Source: CAD feature listing. Evaluate the final solid. Frame: model axes, mm. A direction names the side the tool comes from. Round coordinates to 2 decimals unless told otherwise and drop trailing zeros. Order: outer loops, then holes, each group sorted by start corner. A loop starts at its lowest first (then second) coordinate and runs counter-clockwise, first axis right, second up. Notation, with made-up numbers: (87.25, 89) - (142.25, 89) arc R33 cw to (142.25, 121) - close; hole circle Ø3 at (-35, -14.75). An arc over 180 degrees is marked (long way). Return JSON: item names as keys, results as strings. Group by question number.
1) Mould query, pull axis X, two halves, no side actions, for faces 3 (the cylindrical face through (0.633, 0.493, 2.852)), 4 (the flat face through (0, 0.5, 0)), 5 (the flat face through (0, 4.5, 0)). Classes: pulls with the +X half, pulls with the -X half, needs draft (parallel to the pull), parting line crosses it, or undercut.
2) Section A-A, the plane z = 0. Return loops of the section in (x, y) (3 decimals).
3) Contact query for flat-ended pins moving along their axis: P1, Ø0.6, axis at x = 1.5, y = 0.5, coming from the +Z side; P2, Ø1.5, axis at y = 2.5, z = 2, coming from the +X side; P3, Ø0.6, axis at x = 1.5, y = 0, coming from the -Z side. Output: stop coordinate, or through.
4) Section D-D, the plane z = -2.15. Return loops of the section in (x, y).
5) Ray query, line 1 (Y direction, x = 2.15, z = 1.35); line 2 (Y direction, x = 1.85, z = 0); line 3 (Z direction, x = -1.6, y = 0.3). Return the intervals inside material, ascending. Write a range as from..to.
6) Section C-C, the plane y = 3.7. Return loops of the section in (x, z) (3 decimals).
7) Section B-B, the plane x = 0. Return loops of the section in (y, z) (3 decimals), plus the area to 3 significant figures.
8) Access query for faces 1 (the flat face through (-1.3, 0, -1.3)), 2 (the flat face through (-1, 1, -2)). Directions: +Z, -Z, +X, -X, +Y, -Y. A direction counts if a zero-diameter tool reaches every point of the face in a straight line with its end or side. Return the directions, or none.
Autodesk Inventor part; units mm, degrees
ref_plane "YZ Plane" through (0, 0, 0) normal (1, 0, 0) x (0, 1, 0)
ref_plane "XZ Plane" through (0, 0, 0) normal (0, 1, 0) x (-1, 0, 0)
ref_plane "XY Plane" through (0, 0, 0) normal (0, 0, 1) x (1, 0, 0)
sketch "Sketch1" plane through (0, 0, 0) normal (0, 1, 0) x (-1, 0, 0)
  circle A0 centre (0, 0) radius 2.921
  dimension "d0" = 5.842
extrude "Extrusion1" add sketch "Sketch1" along normal blind 1
sketch "Sketch2" plane through (0, 1, 0) normal (0, 1, 0) x (1, 0, 0)
  circle A0 centre (0, 0) radius 1.905
  dimension "d3" = 3.81
extrude "Extrusion2" add sketch "Sketch2" along normal blind 3.5
sketch "Sketch3" plane through (0, 0, 0) normal (0, -1, 0) x (1, 0, 0)
  line L0 (0, 1.905) -> (-1, 1.905)
  line L1 (-1, -1.905) -> (1, -1.905)
  line L2 (1, 1.905) -> (0, 1.905)
  line L3 (-1.905, 0) -> (-1.905, -1)
  line L4 (1.905, -1) -> (1.905, 1)
  line L5 (-1.905, 0) -> (-1.905, 1)
  line L6 (-1.905, 1) -> (-1, 1)
  line L7 (1, 1) -> (1.905, 1)
  line L8 (1, -1.905) -> (1, -1)
  line L9 (1, 1) -> (1, 1.905)
  line L10 (-1.905, -1) -> (-1, -1)
  line L11 (1, -1) -> (1.905, -1)
  line L12 (-1, 1.905) -> (-1, 1)
  line L13 (-1, -1) -> (-1, -1.905)
  point P0 (0, 0)
  dimension "d7" = 1
  dimension "d8" = 3.81
  dimension "d9" = 2
  dimension "d10" = 3.81
  dimension "d11" = 1
  dimension "d12" = 3.81
  dimension "d13" = 2
  dimension "d15" = 1
extrude "Extrusion3" cut sketch "Sketch3" against normal blind 0.5
properties part number "armscrew" material "Iron, Gray"
Geometry check:
{
 "1": {"face 3": "parting line crosses it", "face 4": "undercut", "face 5": "needs draft"},
 "2": {"outline": "(-2.921, 0) - (-1.905, 0) - (-1.905, 0.5) - (1.905, 0.5) - (1.905, 0) - (2.921, 0) - (2.921, 1) - (1.905, 1) - (1.905, 4.5) - (-1.905, 4.5) - (-1.905, 1) - (-2.921, 1) - close"},
 "3": {"P1": "z = 2.66", "P2": "x = 1.44", "P3": "z = -2.66"},
 "4": {"outline": "(-1.98, 0) - (1.98, 0) - (1.98, 1) - (-1.98, 1) - close"},
 "5": {"line 1": "0..1", "line 2": "0.5..4.5", "line 3": "-2.44..-1, 1..2.44"},
 "6": {"outline": "circle Ø3.81 at (0, 0)"},
 "7": {"outline": "(0, -2.921) - (1, -2.921) - (1, -1.905) - (4.5, -1.905) - (4.5, 1.905) - (1, 1.905) - (1, 2.921) - (0, 2.921) - (0, 1.905) - (0.5, 1.905) - (0.5, -1.905) - (0, -1.905) - close", "area": "17.3 mm2"},
 "8": {"face 1": "+Z, -Z, +X, -X, -Y", "face 2": "+Y"}
}
